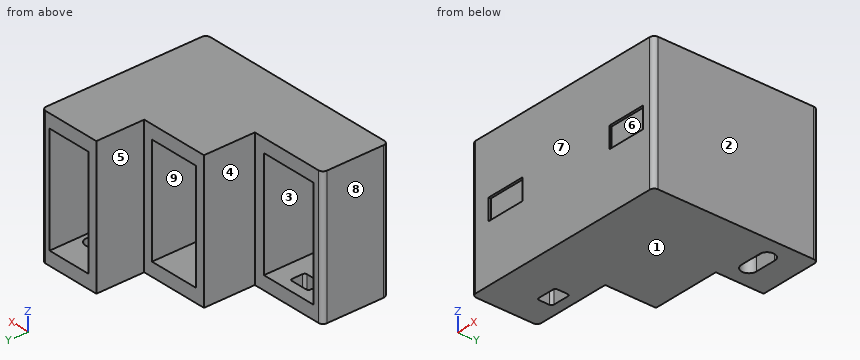
from build123d import *

# Parameters (mm, degrees)
EXTRUDE_1_DEPTH      = 90
SKETCH_2_W           = 38
SKETCH_2_H           = 72
CUT_EXTRUDE_1_DEPTH  = 36
SKETCH_4_W           = 34
SKETCH_4_H           = 72
CUT_EXTRUDE_3_DEPTH  = 70
SKETCH_5_W           = 30
SKETCH_5_H           = 72
CUT_EXTRUDE_4_DEPTH  = 102
SKETCH_7_W           = 26
SKETCH_7_H           = 14
CUT_EXTRUDE_6_DEPTH  = 1.5
FILLET_2_R           = 3
CUT_EXTRUDE_11_DEPTH = 9.5
CUT_EXTRUDE_12_DEPTH = 9.5


with BuildPart() as part:
    # 草图1 → 凸台-拉伸1 (new body)
    with BuildSketch(Plane.XY):
        Polygon((-70, 0), (70, 0), (70, 110), (28, 110), (28, 78), (-18, 78), (-18, 44), (-70, 44), align=None)
    extrude(amount=EXTRUDE_1_DEPTH)

    # 草图2 → 切除-拉伸1 (cut)
    with BuildSketch(Plane(origin=(0, 44, 0), x_dir=(1, 0, 0), z_dir=(0, 1, 0))):
        with Locations((-44, -45)):
            Rectangle(SKETCH_2_W, SKETCH_2_H)
    extrude(amount=-CUT_EXTRUDE_1_DEPTH, mode=Mode.SUBTRACT)

    # 草图4 → 切除-拉伸3 (cut)
    with BuildSketch(Plane(origin=(0, 78, 0), x_dir=(1, 0, 0), z_dir=(0, 1, 0))):
        with Locations((5, -45)):
            Rectangle(SKETCH_4_W, SKETCH_4_H)
    extrude(amount=-CUT_EXTRUDE_3_DEPTH, mode=Mode.SUBTRACT)

    # 草图5 → 切除-拉伸4 (cut)
    with BuildSketch(Plane(origin=(0, 110, 0), x_dir=(1, 0, 0), z_dir=(0, 1, 0))):
        with Locations((49, -45)):
            Rectangle(SKETCH_5_W, SKETCH_5_H)
    extrude(amount=-CUT_EXTRUDE_4_DEPTH, mode=Mode.SUBTRACT)

    # 草图7 → 切除-拉伸6 (cut)
    with BuildSketch(Plane(origin=(0, 0, 0), x_dir=(1, 0, 0), z_dir=(0, 1, 0))):
        with Locations((-44, -45)):
            Rectangle(SKETCH_7_W, SKETCH_7_H)
        with Locations((49, -45)):
            Rectangle(SKETCH_7_W, SKETCH_7_H)
    extrude(amount=CUT_EXTRUDE_6_DEPTH, mode=Mode.SUBTRACT)

    # 圆角2
    fillet_2_edges = [part.edges().sort_by_distance(p)[0] for p in [
        (-70, 44, 45),
        (70, 110, 45),
        (70, 0, 45),
        (-70, 0, 45),
    ]]
    fillet(fillet_2_edges, radius=FILLET_2_R)

    # 草图12 → 切除-拉伸11 (cut)
    with BuildSketch(Plane.XY):
        with BuildLine():
            Line((-49.5, 27), (-38.5, 27))
            ThreePointArc((-38.5, 27), (-37.439339828, 27.439339828), (-37, 28.5))
            Line((-37, 28.5), (-37, 35.5))
            ThreePointArc((-37, 35.5), (-37.439339828, 36.560660172), (-38.5, 37))
            Line((-38.5, 37), (-49.5, 37))
            ThreePointArc((-49.5, 37), (-50.560660172, 36.560660172), (-51, 35.5))
            Line((-51, 35.5), (-51, 28.5))
            ThreePointArc((-51, 28.5), (-50.560660172, 27.439339828), (-49.5, 27))
        make_face()
    extrude(amount=CUT_EXTRUDE_11_DEPTH, mode=Mode.SUBTRACT)

    # 草图13 → 切除-拉伸12 (cut)
    with BuildSketch(Plane.XY):
        with BuildLine():
            Line((42, 83), (56, 83))
            ThreePointArc((56, 83), (61, 88), (56, 93))
            Line((56, 93), (42, 93))
            ThreePointArc((42, 93), (37, 88), (42, 83))
        make_face()
    extrude(amount=CUT_EXTRUDE_12_DEPTH, mode=Mode.SUBTRACT)


solid = part.part
For this review, take the finished solid that the model builds, in its own axes (mm). Face numbers are marked on the shaded views. A direction names the side the tool comes from. Round coordinates to 2 decimals unless told otherwise and drop trailing zeros. Loops run counter-clockwise (first coordinate to the right, second up) from the corner with the lowest first, then second, coordinate; pieces in that order, holes last. Notation, with made-up numbers: (13.5, 21) - (65.5, 21) arc R23 cw to (65.5, 39) - close; hole circle Ø7 at (41.5, 73). An arc over 180 degrees is marked (long way). One line per question, with ' | ' between items.
Q1. The part is to be moulded in two halves that separate along X. For the marked faces 1, 2, 3 and 4, say which applies: released by +X, released by -X, zero draft, split by the parting line, or undercut.
Taken from the geometry:
face 1: zero draft | face 2: released by +X | face 3: undercut | face 4: released by -X
Q2. Take a section at C-C (y = 103). Give the boundary of the cut face in (x, z), and give its area (3 significant figures).
Taken from the geometry:
outline: (28, 0) - (70, 0) - (70, 90) - (28, 90) - close; hole (34, 9) - (64, 9) - (64, 81) - (34, 81) - close | area: 1,620 mm²
Q3. Take a section at B-B (z = 70.5). Give the boundary of the cut face in (x, y), and give its area (3 significant figures).
Taken from the geometry:
outline: (-70, 3) arc R3 ccw to (-67, 0) - (67, 0) arc R3 ccw to (70, 3) - (70, 107) arc R3 ccw to (67, 110) - (64, 110) - (64, 8) - (34, 8) - (34, 110) - (28, 110) - (28, 78) - (22, 78) - (22, 8) - (-12, 8) - (-12, 78) - (-18, 78) - (-18, 44) - (-25, 44) - (-25, 8) - (-63, 8) - (-63, 44) - (-67, 44) arc R3 ccw to (-70, 41) - close | area: 3,680 mm²
Q4. Take a section at A-A (y = 88). Give the boundary of the cut face in (x, z), and give its area (3 significant figures).
Taken from the geometry:
outline: (28, 0) - (37, 0) - (37, 9) - (34, 9) - (34, 81) - (64, 81) - (64, 9) - (61, 9) - (61, 0) - (70, 0) - (70, 90) - (28, 90) - close | area: 1,400 mm²
Q5. Tool access review of the marked faces 5, 6, 7, 8 and 9: name each direction out of +Z, -Z, +X, -X, +Y, -Y from which nothing blocks a thin tool from reaching the whole face with its end or side.
Taken from the geometry:
face 5: +Z, -Z, -X, +Y | face 6: -Y | face 7: +Z, -Z, +X, -X, -Y | face 8: +Z, -Z, -X, +Y, -Y | face 9: +Y
Q6. For line 1 along X through (y, z) = (71.5, 27); line 2 along X through (y, z) = (34.5, 10); line 3 along Z through (x, y) = (-32.5, 16), list the stretches that pass through material, from the lowest coordinate up. Write a range as [from, to].
Taken from the geometry:
line 1: x = [-18, -12], [22, 34], [64, 70] | line 2: x = [-70, -63], [-25, -12], [22, 34], [64, 70] | line 3: z = [0, 9], [81, 90]
Q7. For pin 1 (1.2 mm diameter, centred on y = 0.5, z = 44.5, fed in from +X); pin 2 (7 mm diameter, centred on x = -45, z = 3, fed in from +Y); pin 3 (16 mm diameter, centred on y = 97, z = 60.5, fed in from -X), all flat-tipped, find the tip position at first contact; note any pin that passes through.
Taken from the geometry:
pin 1: stops at x = 69.32 | pin 2: stops at y = 44 | pin 3: stops at x = 28
Q8. Take a section at D-D (y = 64.5). Give the boundary of the cut face in (x, z), and give its area (3 significant figures).
Taken from the geometry:
outline: (-18, 0) - (70, 0) - (70, 90) - (-18, 90) - close; hole (-12, 9) - (22, 9) - (22, 81) - (-12, 81) - close; hole (34, 9) - (64, 9) - (64, 81) - (34, 81) - close | area: 3,310 mm²
